Source: CAD feature listing. Evaluate the final solid. Frame: model axes, mm. A direction names the side the tool comes from. Round coordinates to 2 decimals unless told otherwise and drop trailing zeros. Order: outer loops, then holes, each group sorted by start corner. A loop starts at its lowest first (then second) coordinate and runs counter-clockwise, first axis right, second up. Notation, with made-up numbers: (7.5, 75.25) -> (25.5, 75.25) arc R6 ccw to (25.5, 85.25) -> close; hole circle Ø9 at (1, 53.5). An arc over 180 degrees is marked (long way). Write item = value, one per line. Start each with the question number.
(1) Cut plane A-A on x = 216. Return the cut outline in (y, z).
(2) Cut plane D-D on x = 109.5. Return the cut outline in (y, z).
(3) Cut plane C-C on x = -212. Return the cut outline in (y, z).
(4) Ray query, line 1 (Z direction, x = -102.5, y = -36.5); line 2 (Z direction, x = -225, y = -42). Return the intervals inside material, ascending.
(5) Reachability of faces 1 (the face through (223, -27, -575)), 2 (the face through (-241.94, -23.82, 562.33)), 3 (the face through (206.325, -13.86, -562.325)) from +Z, -Z, +X, -X, +Y, -Y: full face, straight path, thin tool, end or side. Return the list, or none.
(6) Cut plane B-B on y = -38. Return the cut outline in (x, z).
(7) Contact query for flat-ended pins moving along their axis: pin 1 Ø15 at (x, y) = (-60, -21.5) entering from -Z; pin 2 Ø3 at (x, y) = (-121, -32.5) entering from +Z. Output: stop coordinate, or through.
from build123d import *

# Parameters (mm, degrees)
F0_W     = 500
F0_H     = 1100
F1_DEPTH = 50
F2_R     = 21.310821
F3_DEPTH = 25
F4_R     = 21.289227
F5_DEPTH = 25


with BuildPart() as f1:
    # F0 (on Front) → F1 (new body)
    with BuildSketch(Plane.XZ):
        Rectangle(F0_W, F0_H)
    extrude(amount=F1_DEPTH)

    # F2 (on face) → F3 (join)
    with BuildSketch(Plane.XY.offset(550)):
        with Locations((-220.649317, -24.756737)):
            Circle(F2_R)
    extrude(amount=F3_DEPTH)

    # F4 (on face) → F5 (join)
    with BuildSketch(Plane(origin=(0, 0, -550), x_dir=(1, 0, 0), z_dir=(0, 0, -1))):
        with Locations((223.219097, 26.814517)):
            Circle(F4_R)
    extrude(amount=F5_DEPTH)


solid = f1.part
Evaluation:
q1.outline = (-50, -550) -> (-46.84, -550) -> (-46.84, -575) -> (-6.79, -575) -> (-6.79, -550) -> (0, -550) -> (0, 550) -> (-50, 550) -> close
q2.outline = (-50, -550) -> (0, -550) -> (0, 550) -> (-50, 550) -> close
q3.outline = (-50, -550) -> (0, -550) -> (0, 550) -> (-5.28, 550) -> (-5.28, 575) -> (-44.23, 575) -> (-44.23, 550) -> (-50, 550) -> close
q4.line_1 = -550 to 550
q4.line_2 = -550 to 575
q5.face_1 = -Z, +X, -X, +Y, -Y
q5.face_2 = +Z
q5.face_3 = -Z
q6.outline = (-250, -550) -> (205.11, -550) -> (205.11, -575) -> (241.33, -575) -> (241.33, -550) -> (250, -550) -> (250, 550) -> (-203.95, 550) -> (-203.95, 575) -> (-237.35, 575) -> (-237.35, 550) -> (-250, 550) -> close
q7.pin_1 = -550
q7.pin_2 = 550
